Design review of the part built by this model. Coordinates are the model's own, in mm. Give positions to 0.01 mm unless a question says otherwise; leave off trailing zeros. Write each loop counter-clockwise with the first axis right and the second up, starting at its lowest first coordinate (ties: lowest second). Pieces come first, ordered by that corner, then holes. Notation, with made-up numbers: (-8, 68) - (-4, 68) arc R24 ccw to (-4, 90) - close; hole circle Ø6 at (39.5, 85.5). An arc over 180 degrees is marked (long way). Use a Markdown table: item, result. Add a question column.
```python
from build123d import *

# Parameters (mm, degrees)
SKETCH4_R           = 11.95
SKETCH4_R_2         = 6.65
SKETCH4_R_3         = 5.6
SKETCH4_R_4         = 6
SKETCH4_W           = 20.218579234
SKETCH4_H           = 37
SKETCH4_W_2         = 13.5
SKETCH4_H_2         = 28.1
BOSS_EXTRUDE1_DEPTH = 1.6


with BuildPart() as part:
    # Sketch4 → Boss-Extrude1 (new body)
    with BuildSketch(Plane(origin=(0, 0, 0), x_dir=(1, 0, 0), z_dir=(0, 1, 0))):
        with BuildLine():
            Line((-60.547420146, 63.390203379), (394.452579854, 63.390203379))
            Line((394.452579854, 63.390203379), (396.952579854, 63.390203379))
            Line((396.952579854, 63.390203379), (396.952579854, -46.609796621))
            ThreePointArc((396.952579854, -46.609796621), (395.48811376, -50.145330527), (391.952579854, -51.609796621))
            Line((391.952579854, -51.609796621), (-60.547420146, -51.609796621))
            Line((-60.547420146, -51.609796621), (-63.047420146, -51.609796621))
            Line((-63.047420146, -51.609796621), (-63.047420146, 63.390203379))
            Line((-63.047420146, 63.390203379), (-60.547420146, 63.390203379))
        make_face()
        with Locations(Location((54.9, 29.690203379, 0), (0, 0, 270))):
            Circle(SKETCH4_R, mode=Mode.SUBTRACT)
        with Locations(Location((102.75, 30.240203379, 0), (0, 0, 270))):
            Circle(SKETCH4_R_2, mode=Mode.SUBTRACT)
        with Locations(Location((147.75, 30.240203379, 0), (0, 0, 270))):
            Circle(SKETCH4_R_2, mode=Mode.SUBTRACT)
        with Locations(Location((184.9, 30.790203379, 0), (0, 0, 270))):
            Circle(SKETCH4_R_3, mode=Mode.SUBTRACT)
        with Locations(Location((-18.9, -18.109796621, 0), (0, 0, 270))):
            Circle(SKETCH4_R_4, mode=Mode.SUBTRACT)
        with Locations(Location((8.7, -18.109796621, 0), (0, 0, 270))):
            Circle(SKETCH4_R_4, mode=Mode.SUBTRACT)
        with Locations(Location((26.45, -18.109796621, 0), (0, 0, 270))):
            Circle(SKETCH4_R_4, mode=Mode.SUBTRACT)
        with Locations(Location((44.2, -18.109796621, 0), (0, 0, 270))):
            Circle(SKETCH4_R_4, mode=Mode.SUBTRACT)
        with Locations(Location((61.95, -18.109796621, 0), (0, 0, 270))):
            Circle(SKETCH4_R_4, mode=Mode.SUBTRACT)
        with Locations(Location((79.7, -18.109796621, 0), (0, 0, 270))):
            Circle(SKETCH4_R_4, mode=Mode.SUBTRACT)
        with Locations(Location((97.45, -18.109796621, 0), (0, 0, 270))):
            Circle(SKETCH4_R_4, mode=Mode.SUBTRACT)
        with Locations(Location((115.2, -18.109796621, 0), (0, 0, 270))):
            Circle(SKETCH4_R_4, mode=Mode.SUBTRACT)
        with Locations(Location((132.95, -18.109796621, 0), (0, 0, 270))):
            Circle(SKETCH4_R_4, mode=Mode.SUBTRACT)
        with Locations(Location((150.7, -18.109796621, 0), (0, 0, 270))):
            Circle(SKETCH4_R_4, mode=Mode.SUBTRACT)
        with Locations(Location((168.45, -18.109796621, 0), (0, 0, 270))):
            Circle(SKETCH4_R_4, mode=Mode.SUBTRACT)
        with Locations(Location((186.2, -18.109796621, 0), (0, 0, 270))):
            Circle(SKETCH4_R_4, mode=Mode.SUBTRACT)
        with Locations(Location((203.95, -18.109796621, 0), (0, 0, 270))):
            Circle(SKETCH4_R_4, mode=Mode.SUBTRACT)
        with Locations(Location((221.7, -18.109796621, 0), (0, 0, 270))):
            Circle(SKETCH4_R_4, mode=Mode.SUBTRACT)
        with Locations(Location((239.45, -18.109796621, 0), (0, 0, 270))):
            Circle(SKETCH4_R_4, mode=Mode.SUBTRACT)
        with Locations(Location((257.2, -18.109796621, 0), (0, 0, 270))):
            Circle(SKETCH4_R_4, mode=Mode.SUBTRACT)
        with Locations(Location((274.95, -18.109796621, 0), (0, 0, 270))):
            Circle(SKETCH4_R_4, mode=Mode.SUBTRACT)
        with Locations(Location((292.7, -18.109796621, 0), (0, 0, 270))):
            Circle(SKETCH4_R_4, mode=Mode.SUBTRACT)
        with Locations(Location((310.45, -18.109796621, 0), (0, 0, 270))):
            Circle(SKETCH4_R_4, mode=Mode.SUBTRACT)
        with Locations(Location((328.2, -18.109796621, 0), (0, 0, 270))):
            Circle(SKETCH4_R_4, mode=Mode.SUBTRACT)
        with Locations(Location((345.95, -18.109796621, 0), (0, 0, 270))):
            Circle(SKETCH4_R_4, mode=Mode.SUBTRACT)
        with Locations(Location((363.7, -18.109796621, 0), (0, 0, 270))):
            Circle(SKETCH4_R_4, mode=Mode.SUBTRACT)
        with Locations((-18.6, 30.690203379)):
            Rectangle(SKETCH4_W, SKETCH4_H, mode=Mode.SUBTRACT)
        with Locations((12.4, 30.690203379)):
            Rectangle(SKETCH4_W, SKETCH4_H, mode=Mode.SUBTRACT)
        with Locations((241.15, 32.073143277)):
            Rectangle(SKETCH4_W_2, SKETCH4_H_2, mode=Mode.SUBTRACT)
        with Locations((221.15, 32.073143277)):
            Rectangle(SKETCH4_W_2, SKETCH4_H_2, mode=Mode.SUBTRACT)
        with Locations((261.15, 32.073143277)):
            Rectangle(SKETCH4_W_2, SKETCH4_H_2, mode=Mode.SUBTRACT)
        with Locations((281.15, 32.073143277)):
            Rectangle(SKETCH4_W_2, SKETCH4_H_2, mode=Mode.SUBTRACT)
        with Locations((301.15, 32.073143277)):
            Rectangle(SKETCH4_W_2, SKETCH4_H_2, mode=Mode.SUBTRACT)
        with Locations((321.15, 32.073143277)):
            Rectangle(SKETCH4_W_2, SKETCH4_H_2, mode=Mode.SUBTRACT)
    extrude(amount=BOSS_EXTRUDE1_DEPTH)


solid = part.part
```
(1) Mouldability with a two-part tool opening along X and no side actions: class faces 1 (the face through (287.38, 0.79, 20.88)), 2 (the face through (170, 0, -7)) as +X half, -X half, draft (parallel to the pull), parting line (faces both ways), or undercut.
(2) Add section A-A (x = 345.95). State the section outline as (y, z) points, and give its area (3 significant figures).
(3) Add section D-D (x = 221.7). State the section outline as (y, z) points.
(4) Add section B-B (x = -18.9). State the section outline as (y, z) points, and give its area (3 significant figures).
(5) For line 1 along Z through (x, y) = (274.95, 0.85); line 2 along Z through (x, y) = (256.5, 0.85); line 3 along Z through (x, y) = (-9.5, 1.4), list the stretches that pass through material, from the lowest coordinate up.
(6) Add section C-C (y = 0.8). Count the separate pieces of the cut face and the enclosed holes in it, and give its area (3 significant figures).
Answers follow:
| question | item | result |
|---|---|---|
| 1 | face 1 | undercut |
| 1 | face 2 | draft |
| 2 | outline | (0, -63.39) - (1.6, -63.39) - (1.6, 12.11) - (0, 12.11) - close; (0, 24.11) - (1.6, 24.11) - (1.6, 51.61) - (0, 51.61) - close |
| 2 | area | 165 mm^2 |
| 3 | outline | (0, -63.39) - (1.6, -63.39) - (1.6, -46.12) - (0, -46.12) - close; (0, -18.02) - (1.6, -18.02) - (1.6, 12.11) - (0, 12.11) - close; (0, 24.11) - (1.6, 24.11) - (1.6, 51.61) - (0, 51.61) - close |
| 4 | outline | (0, -63.39) - (1.6, -63.39) - (1.6, -49.19) - (0, -49.19) - close; (0, -12.19) - (1.6, -12.19) - (1.6, 12.11) - (0, 12.11) - close; (0, 24.11) - (1.6, 24.11) - (1.6, 51.61) - (0, 51.61) - close |
| 4 | area | 106 mm^2 |
| 5 | line 1 | -63.39 to -46.12, -18.02 to 12.11, 24.11 to 51.61 |
| 5 | line 2 | -63.39 to -46.12, -18.02 to 12.15, 24.07 to 51.61 |
| 5 | line 3 | -63.39 to -49.19, -12.19 to 51.61 |
| 6 | separate pieces | 1 |
| 6 | enclosed holes | 34 |
| 6 | area | 45,800 mm^2 |
